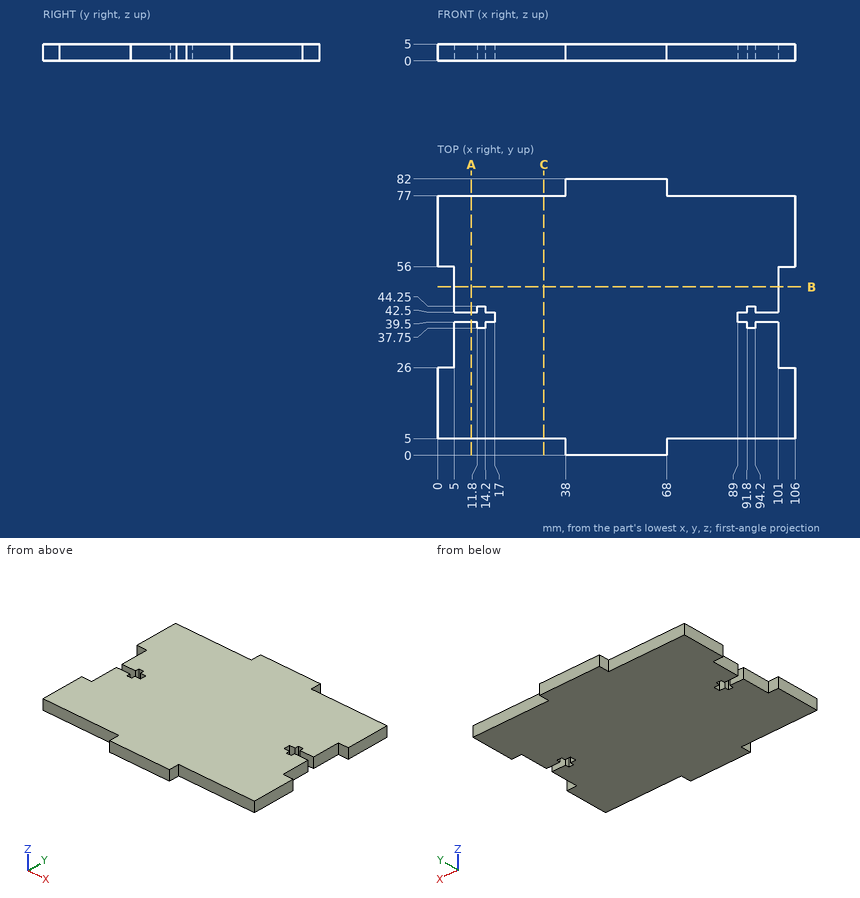
Verification items for this drawing (mm, ordinates from the low corner). Give positions to 0.01 mm unless a question says otherwise; leave off trailing zeros. Loops run counter-clockwise (first coordinate to the right, second up) from the corner with the lowest first, then second, coordinate; pieces in that order, holes last. Notation, with made-up numbers: M 16.25,89.5 L 71.25,89.5 A30 cw 71.25,128.5 Z; hole C -32.5,8 d6. An arc over 180 degrees is marked long. Answer as a JSON object with one key per item and string values. Group by question number.
Q1. Material ranges on line 1 along X through (y, z) = (38, 3.1); line 2 along Y through (x, z) = (93, 1.2); line 3 along Y through (x, z) = (77, 0.95), recorded low to high. Write a range as [from, to].
Q2. Cross-section at A-A on x = 10. Record the cut outline in (y, z).
Q3. Cross-section at C-C on x = 31.5. Record the cut outline in (y, z).
Q4. Cross-section at B-B on y = 50. Record the cut outline in (x, z).
Q5. Go/stop test with flat-tipped pins: P1, Ø0.5, axis at y = 43.5, z = 2.5, coming from the -X side; P2, Ø0.9, axis at y = 38.5, z = 3.5, coming from the +X side; P3, Ø1.5, axis at x = 8.5, z = 3.5, coming from the +Y side. Record where each tip stops, or that it passes through.
Evaluation:
{
 "1": {"line 1": "x = [5, 11.8], [14.2, 91.8], [94.2, 101]", "line 2": "y = [5, 37.75], [44.25, 77]", "line 3": "y = [5, 77]"},
 "2": {"outline": "M 5,0 L 39.5,0 L 39.5,5 L 5,5 Z; M 42.5,0 L 77,0 L 77,5 L 42.5,5 Z"},
 "3": {"outline": "M 5,0 L 77,0 L 77,5 L 5,5 Z"},
 "4": {"outline": "M 5,0 L 101,0 L 101,5 L 5,5 Z"},
 "5": {"P1": "stops at x = 5", "P2": "stops at x = 101", "P3": "stops at y = 77"}
}
